```python
from build123d import *

# Parameters (mm, degrees)
SKETCH1_R           = 50
BOSS_EXTRUDE1_DEPTH = 20
SKETCH2_R           = 30
BOSS_EXTRUDE2_DEPTH = 30
CUT_EXTRUDE1_DEPTH  = 50
CUT_EXTRUDE2_DEPTH  = 10


with BuildPart() as part:
    # Sketch1 → Boss-Extrude1 (new body)
    with BuildSketch(Plane(origin=(0, 0, 0), x_dir=(0, 0, -1), z_dir=(1, 0, 0))):
        Circle(SKETCH1_R)
    extrude(amount=BOSS_EXTRUDE1_DEPTH)

    # Sketch2 → Boss-Extrude2 (add)
    with BuildSketch(Plane(origin=(20, 0, 0), x_dir=(0, 0, -1), z_dir=(1, 0, 0))):
        Circle(SKETCH2_R)
    extrude(amount=BOSS_EXTRUDE2_DEPTH)

    # Sketch3 → Cut-Extrude1 (cut)
    with BuildSketch(Plane.ZY):
        with BuildLine():
            Line((-5.23333009, 16.081894033), (4.76666991, 16.081894033))
            Line((4.76666991, 16.081894033), (4.76666991, 14.222477209))
            ThreePointArc((4.76666991, 14.222477209), (0.247488145, -14.997958182), (-5.23333009, 14.05746265))
            Line((-5.23333009, 14.05746265), (-5.23333009, 16.081894033))
        make_face()
    extrude(amount=-CUT_EXTRUDE1_DEPTH, mode=Mode.SUBTRACT)

    # Sketch4 → Cut-Extrude2 (cut)
    with BuildSketch(Plane.ZY):
        with BuildLine():
            Line((-13.747727085, 6), (-49.638694584, 6))
            ThreePointArc((-49.638694584, 6), (-50, 0), (-49.638694584, -6))
            Line((-49.638694584, -6), (-13.747727085, -6))
            ThreePointArc((-13.747727085, -6), (-15, 0), (-13.747727085, 6))
        make_face()
        with BuildLine():
            ThreePointArc((50, 0), (49.90959191, 3.005434312), (49.638694584, 6))
            Line((49.638694584, 6), (13.747727085, 6))
            ThreePointArc((13.747727085, 6), (15, 0), (13.747727085, -6))
            Line((13.747727085, -6), (49.638694584, -6))
            ThreePointArc((49.638694584, -6), (49.90959191, -3.005434312), (50, 0))
        make_face()
    extrude(amount=-CUT_EXTRUDE2_DEPTH, mode=Mode.SUBTRACT)


solid = part.part
```
Check sheet for the modelled part. Datum: model origin and axes. Units: mm. A direction names the side the tool comes from. Give positions to 0.01 mm unless a question says otherwise; leave off trailing zeros. Order: outer loops, then holes, each group sorted by start corner. A loop starts at its lowest first (then second) coordinate and runs counter-clockwise, first axis right, second up. Notation, with made-up numbers: (-20.5, -6.5) -> (36.5, -6.5) arc R29 cw to (36.5, 25.5) -> close; hole circle Ø2 at (76.25, -13.5). An arc over 180 degrees is marked (long way). Use CSV: the item, a comma, the result in double quotes. Start each with the question number.
1) Material ranges on line 1 (Y direction, x = 23.5, z = 0); line 2 (Y direction, x = 13.5, z = 0); line 3 (Z direction, x = 11.5, y = 0), recorded low to high. Write a range as from..to.
2) Sectioned sample at A-A, the plane y = 0. Record the boundary of the cut face in (x, z), plus the area to 3 significant figures.
3) Sectioned sample at C-C, the plane x = 12. Record the boundary of the cut face in (y, z), plus the area to 3 significant figures.
4) Sectioned sample at D-D, the plane z = 19.5. Record the boundary of the cut face in (x, y).
5) Sectioned sample at B-B, the plane z = 0. Record the boundary of the cut face in (x, y).
6) Set-up check for faces 4 (the face through (50, 14, -6)), 5 (the face through (0, 23, 1)), 6 (the face through (20, -22, -22)), 7 (the face through (10, 0, -32)), 8 (the face through (25, 16.082, 0)): record each of +Z, -Z, +X, -X, +Y, -Y from which the full face is reachable in a straight line by a thin tool's end or side.
7) Mould release check, pull along Z, two halves, no side actions. Record for faces 1 (the face through (9.86, 15.02, -47.69)), 2 (the face through (24.65, -14.977, 0.835)), 3 (the face through (0, -28, 1)): released by +Z, released by -Z, zero draft, split by the parting line, or undercut.
8) Go/stop test with flat-tipped pins: P1, Ø11, axis at x = 4, z = -32, coming from the -Y side; P2, Ø6, axis at y = 2, z = 24, coming from the -X side; P3, Ø10, axis at x = 15.5, y = -20.5, coming from the +Z side. Record where each tip stops, or that it passes through.
Recorded:
1,line 1,"-30..-15, 16.08..30"
1,line 2,"-50..-15, 16.08..50"
1,line 3,"-50..-15, 15..50"
2,outline,"(10, -50) -> (20, -50) -> (20, -30) -> (50, -30) -> (50, -15) -> (10, -15) -> close; (10, 15) -> (50, 15) -> (50, 30) -> (20, 30) -> (20, 50) -> (10, 50) -> close"
2,area,"1,600 mm2"
3,outline,"circle Ø100 at (0, 0); hole (14.06, -5.23) -> (16.08, -5.23) -> (16.08, 4.77) -> (14.22, 4.77) arc R15 ccw (long way) to start"
3,area,"7,130 mm2"
4,outline,"(0, -46.04) -> (20, -46.04) -> (20, -22.8) -> (50, -22.8) -> (50, 22.8) -> (20, 22.8) -> (20, 46.04) -> (0, 46.04) -> (0, 6) -> (10, 6) -> (10, -6) -> (0, -6) -> close"
5,outline,"(0, -50) -> (20, -50) -> (20, -30) -> (50, -30) -> (50, -15) -> (0, -15) -> close; (0, 16.08) -> (50, 16.08) -> (50, 30) -> (20, 30) -> (20, 50) -> (0, 50) -> close"
6,face 4,"+Z, -Z, +X, +Y, -Y"
6,face 5,"+Z, -Z, -X, +Y, -Y"
6,face 6,"+X"
6,face 7,"+Z, -Z, -X"
6,face 8,"+X, -X"
7,face 1,"split by the parting line"
7,face 2,"undercut"
7,face 3,"zero draft"
8,P1,"y = -42.4"
8,P2,"x = 10"
8,P3,"z = 47.54"
